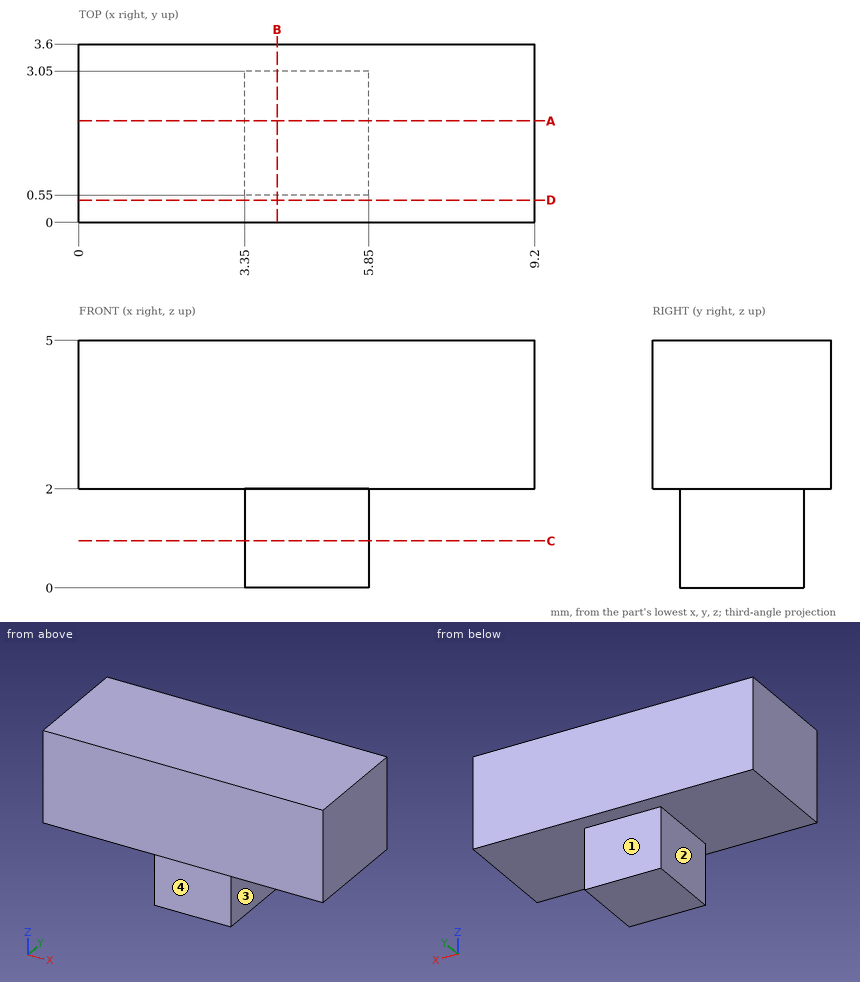
Here's the drawing with two shaded views (mm, measured from the low corner). I have some questions. A direction names the side the tool comes from. Give positions to 0.01 mm unless a question says otherwise; leave off trailing zeros. Write each loop counter-clockwise with the first axis right and the second up, starting at its lowest first coordinate (ties: lowest second). Pieces come first, ordered by that corner, then holes. Notation, with made-up numbers: (10, 52) -> (43, 52) arc R19 cw to (43, 76) -> close; hole circle Ø2 at (-33.75, 86). An arc over 180 degrees is marked (long way). Answer as a JSON object with one key per item and string values. Group by question number.
Item 1: Suppose I cut it at B-B (x = 4). Please give me the cut outline in (y, z).
Item 2: For the marked faces 1, 2, 3 and 4, which set-ups out of +Z, -Z, +X, -X, +Y, -Y let a thin tool reach every point of the face, with its end or its side?
Item 3: Suppose I cut it at C-C (z = 0.95). Please give me the cut outline in (x, y).
Item 4: I'm going to push flat-ended pins straight in: P1, Ø1.5, axis at x = 1.5, y = 2, coming from the -Z side; P2, Ø1.5, axis at y = 0.5, z = 1.5, coming from the +X side; P3, Ø2, axis at y = 1.5, z = 0.5, coming from the -X side; P4, Ø1, axis at x = 4, z = 1, coming from the -Y side. Where does each tip first touch, or does it pass through?
Item 5: Please list where these lines run through material, in increasing order: line 1 (Z direction, x = 2.5, y = 3.4); line 2 (X direction, y = 0.6, z = 1.35); line 3 (Y direction, x = 5.25, z = 1.4). Write a range as [from, to].
Item 6: Suppose I cut it at A-A (y = 2.05). Please give me the cut outline in (x, z), plus the area to 3 significant figures.
Item 7: Suppose I cut it at D-D (y = 0.45). Please give me the cut outline in (x, z).
Findings:
{
 "1": {"outline": "(0, 2) -> (0.55, 2) -> (0.55, 0) -> (3.05, 0) -> (3.05, 2) -> (3.6, 2) -> (3.6, 5) -> (0, 5) -> close"},
 "2": {"face 1": "-Z, +X, -X, +Y", "face 2": "-Z, -X, +Y, -Y", "face 3": "-Z, +X, +Y, -Y", "face 4": "-Z, +X, -X, -Y"},
 "3": {"outline": "(3.35, 0.55) -> (5.85, 0.55) -> (5.85, 3.05) -> (3.35, 3.05) -> close"},
 "4": {"P1": "stops at z = 2", "P2": "stops at x = 9.2", "P3": "stops at x = 3.35", "P4": "stops at y = 0.55"},
 "5": {"line 1": "z = [2, 5]", "line 2": "x = [3.35, 5.85]", "line 3": "y = [0.55, 3.05]"},
 "6": {"outline": "(0, 2) -> (3.35, 2) -> (3.35, 0) -> (5.85, 0) -> (5.85, 2) -> (9.2, 2) -> (9.2, 5) -> (0, 5) -> close", "area": "32.6 mm²"},
 "7": {"outline": "(0, 2) -> (9.2, 2) -> (9.2, 5) -> (0, 5) -> close"}
}
